Source: CAD feature listing. Evaluate the final solid. Frame: model axes, mm. A direction names the side the tool comes from. Give positions to 0.01 mm unless a question says otherwise; leave off trailing zeros. Write each loop counter-clockwise with the first axis right and the second up, starting at its lowest first coordinate (ties: lowest second). Pieces come first, ordered by that corner, then holes. Notation, with made-up numbers: M -27,9 L 31,9 A31 cw 31,38 Z; hole C 41,82 d11. An arc over 180 degrees is marked long. Use CSV: the item, a comma, the result in double quotes. Start each with the question number.
Autodesk Inventor part; units mm, degrees
ref_plane "YZ Plane" through (0, 0, 0) normal (1, 0, 0) x (0, 1, 0)
ref_plane "XZ Plane" through (0, 0, 0) normal (0, 1, 0) x (-1, 0, 0)
ref_plane "XY Plane" through (0, 0, 0) normal (0, 0, 1) x (1, 0, 0)
sketch "Sketch1" plane through (0, 0, 0) normal (1, 0, 0) x (0, 1, 0)
  line L0 (-58, -40) -> (-58, 50)
  line L1 (0, 0) -> (-57.3223, 54.5531) construction
  arc A0 (-28.7141, 16.9733) -> (-18.3732, 27.8392) centre (-23.5426, 22.4053) ccw
  circle A1 centre (0, 0) radius 47 construction
  arc A2 (-38.0949, 46.601) -> (-48.4307, 35.7445) centre (-43.4633, 41.3636) ccw
  circle A3 centre (0, 0) radius 10
  line L2 (-11, -52) -> (14.1774, -52)
  line L3 (-58, 0) -> (-58, -40)
  line L4 (0, 0) -> (0, -52) construction
  line L5 (-58, -40) -> (-23, -52.739)
  circle A4 centre (0, 0) radius 50 construction
  arc A5 (22.2788, -50.2857) -> (0, 55) centre (0, 0) ccw
  arc A6 (-53, 55) -> (-58, 50) centre (-53, 50) ccw
  line L6 (-11, 54) -> (-11, 50)
  line L7 (-12, 49) -> (-22, 49)
  line L8 (-23, 50) -> (-23, 54)
  line L9 (-53, 55) -> (-24, 55)
  line L10 (-10, 55) -> (0, 55)
  arc A7 (-23, 54) -> (-24, 55) centre (-24, 54) ccw
  arc A8 (-10, 55) -> (-11, 54) centre (-10, 54) ccw
  arc A9 (-12, 49) -> (-11, 50) centre (-12, 50) ccw
  arc A10 (-23, 50) -> (-22, 49) centre (-22, 50) ccw
  arc A11 (14.1774, -52) -> (22.2788, -50.2857) centre (14.1774, -32) ccw
  line L11 (-23, -49.5) -> (-23, -52.739)
  line L12 (-11, -52) -> (-11, -49.5)
  line L13 (-11.5, -49) -> (-22.5, -49)
  arc A12 (-11, -49.5) -> (-11.5, -49) centre (-11.5, -49.5) ccw
  arc A13 (-22.5, -49) -> (-23, -49.5) centre (-22.5, -49.5) ccw
  line L14 (-38.5, 46.9864) -> (-18.3732, 27.8392)
  line L15 (-48.8316, 36.1262) -> (-28.7141, 16.9733)
  point P0 (-57.7919, 55)
  point P1 (-58, 55)
  point P2 (-25.2108, 39.6663)
  point P3 (17.9165, -52)
  point P4 (-23, 55)
  point P5 (-11, 52)
  dimension "d4" = 94
  dimension "d3" = 32.5
  dimension "d6" = 15
  dimension "d7" = 15
  dimension "d9" = 20
  dimension "d13" = 52
  dimension "d20" = 100
  dimension "d31" = 55
  dimension "d34" = 58
  dimension "d52" = 5
  dimension "d54" = 47
  dimension "d56" = 1
  dimension "d59" = 20
  dimension "d60" = 12
  dimension "d61" = 6
  dimension "d65" = 0.5
  dimension "d69" = 60
  dimension "d72" = 95
  dimension "d74" = 110
  dimension "d75" = 3
  dimension "d76" = 12
  dimension "d77" = 35
extrude "Extrusion4" add sketch "Sketch1" along normal blind 6
fillet "Fillet1" radius 5 1 edges at (3, -58, -40)
fillet "Fillet2" radius 1.5 2 edges at (3, -23, -52.739) (3, -11, -52)
properties part number "MidFlange27130914"
Item 1: Material intervals for probe 1 along Z at (x, y) = (3, 0); probe 2 along Y at (x, z) = (0.35, 7.5); probe 3 along Y at (x, z) = (4.95, 30.5), sorted ascending.
Item 2: Section D-D (z = -20). Return the cut outline in (x, y).
Item 3: Section C-C (y = -40). Return the cut outline in (x, z), plus the area to 3 significant figures.
Item 4: Contact query for flat-ended pins moving along their axis: pin 1 Ø1.8 at (x, y) = (4, -16.5) entering from -Z; pin 2 Ø1 at (x, z) = (4, -12.5) entering from +Y; pin 3 Ø1.2 at (x, z) = (2.5, -50) entering from +Y. Output: stop coordinate, or through.
Item 5: Set-up query: faces 1 (the flat face through (2.96, -38.71, 26.49)), 2 (the flat face through (3, -17, -49)), 3 (the flat face through (3, -23, 52)). Return all of +Z, -Z, +X, -X, +Y, -Y with unobstructed straight access to the full face (end or side cutting, diameter ignored); none if empty.
Item 6: Section B-B (x = 4.35). Return the cut outline in (y, z), plus the area to 3 significant figures.
Item 7: Pull-direction query (Z, two-part tool) for faces 4 (the flat face through (3, -11, 52)), 5 (the flat face through (3, 2, -52)), 6 (the flat face through (3, -28, 37)), 7 (the cylindrical face through (2.96, 53.58, 12.41)); classes: released by +Z, released by -Z, zero draft, split by the parting line, or undercut.
Item 8: Section A-A (z = 0). Return the cut outline in (x, y), plus the area to 3 significant figures.
Output values:
1,probe 1,"z = -52 to -10, 10 to 55"
1,probe 2,"y = -58 to -6.61, 6.61 to 54.49"
1,probe 3,"y = -58 to -42.92, -21.17 to 45.77"
2,outline,"M 0,-58 L 6,-58 L 6,51.23 L 0,51.23 Z"
3,outline,"M 0,-46.55 L 6,-46.55 L 6,27.72 L 0,27.72 Z; M 0,48.02 L 6,48.02 L 6,55 L 0,55 Z"
3,area,"488 mm2"
4,pin 1,"stops at z = -49"
4,pin 2,"stops at y = 53.67"
4,pin 3,"stops at y = 24.18"
5,face 1,"+X, -X"
5,face 2,"-Z, +X, -X"
5,face 3,"+Z, +X, -X"
6,outline,"M -58,-36.5 A5 ccw -54.71,-41.2 L -25.01,-52.01 A1.5 ccw -23,-50.6 L -23,-49.5 A0.5 cw -22.5,-49 L -11.5,-49 A0.5 cw -11,-49.5 L -11,-50.5 A1.5 ccw -9.5,-52 L 14.18,-52 A20 ccw 22.28,-50.29 A55 ccw 0,55 L -10,55 A1 ccw -11,54 L -11,50 A1 cw -12,49 L -22,49 A1 cw -23,50 L -23,54 A1 ccw -24,55 L -53,55 A5 ccw -58,50 Z; hole M -48.43,35.74 L -28.71,16.97 A7.5 ccw -18.37,27.84 L -38.09,46.6 A7.5 ccw long Z; hole C 0,0 d20"
6,area,"9,700 mm2"
7,face 4,"zero draft"
7,face 5,"released by -Z"
7,face 6,"undercut"
7,face 7,"split by the parting line"
8,outline,"M 0,-58 L 6,-58 L 6,-10 L 0,-10 Z; M 0,10 L 6,10 L 6,55 L 0,55 Z"
8,area,"558 mm2"
